Can you work these out from the model? Positions are in its coordinate system, mm. Face numbers are marked on the shaded views. A direction names the side the tool comes from. Round coordinates to 2 decimals unless told otherwise and drop trailing zeros. Loops run counter-clockwise (first coordinate to the right, second up) from the corner with the lowest first, then second, coordinate; pieces in that order, holes last.
from build123d import *

# Parameters (mm, degrees)
SCHIZZO1_R                   = 1.45
SCHIZZO1_R_2                 = 1.33
ESTRUSIONE_ESTRUSIONE1_DEPTH = 4.02
ESTRUSIONE_ESTRUSIONE2_START = -4.02
SCHIZZO2_R                   = 7.37
SCHIZZO2_R_2                 = 1.45
ESTRUSIONE_ESTRUSIONE2_DEPTH = 5.95
ESTRUSIONE_ESTRUSIONE3_START = -4.02
ESTRUSIONE_ESTRUSIONE3_DEPTH = 6.87
FORO_FILETTATO_M3X0_5_1_D    = 2.5
SCHIZZO6_R                   = 4
TAGLIO_ESTRUSIONE1_DEPTH     = 1.07
SCHIZZO8_R                   = 2.9
TAGLIO_ESTRUSIONE2_DEPTH     = 3
SCHIZZO9_W                   = 0.7
SCHIZZO9_H                   = 1.93
TAGLIO_ESTRUSIONE3_DEPTH     = 4.8
SCHIZZO11_W                  = 0.7
SCHIZZO11_H                  = 1.93
TAGLIO_ESTRUSIONE4_DEPTH     = 4.8
SCHIZZO12_R                  = 1.89
ESTRUSIONE_ESTRUSIONE4_DEPTH = 2.03
SCHIZZO13_R                  = 1.89
ESTRUSIONE_ESTRUSIONE5_DEPTH = 2.03


with BuildPart() as part:
    # Schizzo1 → Estrusione-Estrusione1 (new body)
    with BuildSketch(Plane.XY):
        with BuildLine():
            Line((13.603470146, -3.75), (23.88, -3.75))
            ThreePointArc((23.88, -3.75), (27.63, 0), (23.88, 3.75))
            Line((23.88, 3.75), (13.603470146, 3.75))
            ThreePointArc((13.603470146, 3.75), (8.460288245, 4.422618389), (3.663046217, 6.395232006))
            ThreePointArc((3.663046217, 6.395232006), (-7.37, 0), (3.663046217, -6.395232006))
            ThreePointArc((3.663046217, -6.395232006), (8.460288245, -4.422618389), (13.603470146, -3.75))
        make_face()
        Circle(SCHIZZO1_R, mode=Mode.SUBTRACT)
        with Locations((9.13, 0)):
            Circle(SCHIZZO1_R_2, mode=Mode.SUBTRACT)
    extrude(amount=ESTRUSIONE_ESTRUSIONE1_DEPTH)

    # Schizzo2 → Estrusione-Estrusione2 (add)
    with BuildSketch(Plane.XY.offset(4.02).offset(ESTRUSIONE_ESTRUSIONE2_START)):
        with Locations(Location((0, 0, 0), (0, 0, 180))):
            Circle(SCHIZZO2_R)
        with Locations(Location((0, 0, 0), (0, 0, 180))):
            Circle(SCHIZZO2_R_2, mode=Mode.SUBTRACT)
    extrude(amount=ESTRUSIONE_ESTRUSIONE2_DEPTH)

    # Schizzo3 → Estrusione-Estrusione3 (add)
    with BuildSketch(Plane.XY.offset(4.02).offset(ESTRUSIONE_ESTRUSIONE3_START)):
        with BuildLine():
            ThreePointArc((22.819672131, -2.627018485), (26.88, 0), (22.819672131, 2.627018485))
            ThreePointArc((22.819672131, 2.627018485), (22, 2.451336878), (21.180327869, 2.627018485))
            ThreePointArc((21.180327869, 2.627018485), (17.12, 0), (21.180327869, -2.627018485))
            ThreePointArc((21.180327869, -2.627018485), (22, -2.451336878), (22.819672131, -2.627018485))
        make_face()
    extrude(amount=ESTRUSIONE_ESTRUSIONE3_DEPTH)

    # Foro filettato M3x0.5-1 (through all)
    with Locations(Plane.XY.offset(6.87)):
        with Locations((24, 0), (20, 0)):
            Hole(FORO_FILETTATO_M3X0_5_1_D / 2)

    # Schizzo6 → Taglio-Estrusione1 (cut)
    with BuildSketch(Plane(origin=(0, 0, 0), x_dir=(-1, 0, 0), z_dir=(0, 0, -1))):
        Circle(SCHIZZO6_R)
    extrude(amount=-TAGLIO_ESTRUSIONE1_DEPTH, mode=Mode.SUBTRACT)

    # Schizzo8 → Taglio-Estrusione2 (cut)
    with BuildSketch(Plane.XY.offset(5.95)):
        Circle(SCHIZZO8_R)
    extrude(amount=-TAGLIO_ESTRUSIONE2_DEPTH, mode=Mode.SUBTRACT)

    # Schizzo9 → Taglio-Estrusione3 (cut)
    with BuildSketch(Plane(origin=(0, 7.37, 0), x_dir=(1, 0, 0), z_dir=(0, 1, 0))):
        with BuildLine():
            ThreePointArc((2.17, -4.02), (4.42, -1.77), (6.67, -4.02))
            Line((6.67, -4.02), (6.67, -5.95))
            Line((6.67, -5.95), (2.17, -5.95))
            Line((2.17, -5.95), (2.17, -4.02))
        make_face()
        with Locations((7.02, -4.985)):
            Rectangle(SCHIZZO9_W, SCHIZZO9_H)
    extrude(amount=-TAGLIO_ESTRUSIONE3_DEPTH, mode=Mode.SUBTRACT)

    # Schizzo11 → Taglio-Estrusione4 (cut)
    with BuildSketch(Plane(origin=(0, -7.37, 0), x_dir=(-1, 0, 0), z_dir=(0, -1, 0))):
        with BuildLine():
            ThreePointArc((2.17, -4.02), (4.42, -1.77), (6.67, -4.02))
            Line((6.67, -4.02), (6.67, -5.95))
            Line((6.67, -5.95), (2.17, -5.95))
            Line((2.17, -5.95), (2.17, -4.02))
        make_face()
        with Locations((7.02, -4.985)):
            Rectangle(SCHIZZO11_W, SCHIZZO11_H)
    extrude(amount=-TAGLIO_ESTRUSIONE4_DEPTH, mode=Mode.SUBTRACT)

    # Schizzo12 → Estrusione-Estrusione4 (add)
    with BuildSketch(Plane(origin=(0, 2.57, 0), x_dir=(1, 0, 0), z_dir=(0, 1, 0))):
        with Locations(Location((4.42, -4.02, 0), (0, 0, 270))):
            Circle(SCHIZZO12_R)
    extrude(amount=ESTRUSIONE_ESTRUSIONE4_DEPTH)

    # Schizzo13 → Estrusione-Estrusione5 (add)
    with BuildSketch(Plane(origin=(0, -2.57, 0), x_dir=(-1, 0, 0), z_dir=(0, -1, 0))):
        with Locations(Location((4.42, -4.02, 0), (0, 0, 90))):
            Circle(SCHIZZO13_R)
    extrude(amount=ESTRUSIONE_ESTRUSIONE5_DEPTH)


solid = part.part
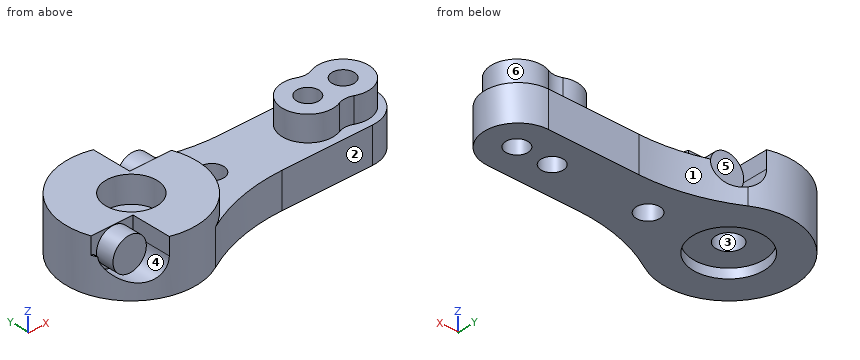
(1) Will these pins go through, and if not, where does the flat tip stop? P1, Ø1.2, axis at x = 19, z = 1.5, coming from the -Y side; P2, Ø3.5, axis at x = 5.5, z = 3.5, coming from the +Y side; P3, Ø2, axis at x = 12, y = -2.5, coming from the +Z side.
Worked answers:
P1: stops at y = -3.75
P2: stops at y = 5.71
P3: stops at z = 4.02
(2) If we section it at C-C, the plane x = 20: List the corners of the cut face in (y, z) for me, then the cut area to 3 significant figures.
Worked answers:
outline: (-3.75, 0) - (-1.25, 0) - (-1.25, 6.87) - (-2.88, 6.87) - (-2.88, 4.02) - (-3.75, 4.02) - close; (1.25, 0) - (3.75, 0) - (3.75, 4.02) - (2.88, 4.02) - (2.88, 6.87) - (1.25, 6.87) - close
area: 29.4 mm2
(3) If we section it at D-D, the plane z = 0.75: List the corners of the cut face in (x, y) for me.
Worked answers:
outline: (3.66, -6.4) arc R20 cw to (13.6, -3.75) - (23.88, -3.75) arc R3.75 ccw to (23.88, 3.75) - (13.6, 3.75) arc R20 cw to (3.66, 6.4) arc R7.37 ccw (long way) to start; hole circle Ø8 at (0, 0); hole circle Ø2.66 at (9.13, 0); hole circle Ø2.5 at (20, 0); hole circle Ø2.5 at (24, 0)
(4) If we mould it in two halves opening along X, with no side actions, what happens to the marked faces 1, 2 and 3? For each: released by +X, released by -X, zero draft, split by the parting line, or undercut.
Worked answers:
face 1: released by +X
face 2: zero draft
face 3: undercut
(5) If I drill on line 1 (Y direction, x = 20, z = 2.5); line 2 (Y direction, x = 0, z = 4.65); line 3 (X direction, y = -0.5, z = 5.5), over which ranges is the centre line in solid material (lowest first)?
Worked answers:
line 1: y = -3.75 to -1.25, 1.25 to 3.75
line 2: y = -7.37 to -2.9, 2.9 to 7.37
line 3: x = -7.35 to -2.86, 2.86 to 7.35, 17.16 to 18.85, 21.15 to 22.85, 25.15 to 26.84
(6) If we section it at A-A, the plane y = 0: State how many separate pieces and enclosed holes the cut face has, then the cut area to 3 significant figures.
Worked answers:
separate pieces: 5
enclosed holes: 0
area: 121 mm2
(7) If we section it at B-B, the plane z = 5.5: List the corners of the cut face in (x, y) for me.
Worked answers:
outline: (-6.91, -2.57) - (-5.6, -2.57) - (-5.6, -4.6) - (-3.24, -4.6) - (-3.24, -2.57) - (-2.17, -2.57) - (-2.17, -7.04) arc R7.37 ccw to (6.91, 2.57) - (5.6, 2.57) - (5.6, 4.6) - (3.24, 4.6) - (3.24, 2.57) - (2.17, 2.57) - (2.17, 7.04) arc R7.37 ccw to start; (21.18, -2.63) arc R2 cw to (22.82, -2.63) arc R2.88 ccw (long way) to (22.82, 2.63) arc R2 cw to (21.18, 2.63) arc R2.88 ccw (long way) to start; hole circle Ø5.8 at (0, 0); hole circle Ø2.5 at (20, 0); hole circle Ø2.5 at (24, 0)
(8) For the marked faces 4, 5 and 6, which set-ups out of +Z, -Z, +X, -X, +Y, -Y let a thin tool reach every point of the face, with its end or its side?
Worked answers:
face 4: -Y
face 5: +Z, +Y
face 6: +Z
